```python
from build123d import *

# Parameters (mm, degrees)
SKETCH1_W           = 79.375
SKETCH1_H           = 82.55
SKETCH1_R           = 32.54375
BOSS_EXTRUDE1_DEPTH = 4.7625
SKETCH2_R           = 1.5875
CUT_EXTRUDE1_DEPTH  = 12.7
SKETCH3_W           = 12.7
SKETCH3_H           = 6.35
CUT_EXTRUDE2_DEPTH  = 10.525
FILLET1_R           = 1.5875


with BuildPart() as part:
    # Sketch1 → Boss-Extrude1 (new body, symmetric)
    with BuildSketch(Plane(origin=(0, 0, 0), x_dir=(1, 0, 0), z_dir=(0, 1, 0))):
        Rectangle(SKETCH1_W, SKETCH1_H)
        Circle(SKETCH1_R, mode=Mode.SUBTRACT)
    extrude(amount=BOSS_EXTRUDE1_DEPTH, both=True)

    # Sketch2 → Cut-Extrude1 (cut)
    with BuildSketch(Plane.ZY.offset(39.6875)):
        with Locations((-22.225, 0)):
            Circle(SKETCH2_R)
        with Locations((22.225, 0)):
            Circle(SKETCH2_R)
    cut_extrude1 = extrude(amount=-CUT_EXTRUDE1_DEPTH, mode=Mode.SUBTRACT)

    # Mirror1: Cut-Extrude1 across plane
    add(cut_extrude1.mirror(Plane(origin=(0, 0, 0), x_dir=(0, 0, 1), z_dir=(1, 0, 0))), mode=Mode.SUBTRACT)

    # Sketch3 → Cut-Extrude2 (cut, through all)
    with BuildSketch(Plane(origin=(34.925, 4.7625, 0), x_dir=(0, 0, -1), z_dir=(0, -1, 0))):
        with Locations((34.925, 1.5875)):
            Rectangle(SKETCH3_W, SKETCH3_H)
    extrude(amount=CUT_EXTRUDE2_DEPTH, mode=Mode.SUBTRACT)

    # Fillet1
    fillet1_edges = [part.edges().sort_by_distance(p)[0] for p in [
        (33.3375, 0, -28.575),
    ]]
    fillet(fillet1_edges, radius=FILLET1_R)


solid = part.part
```
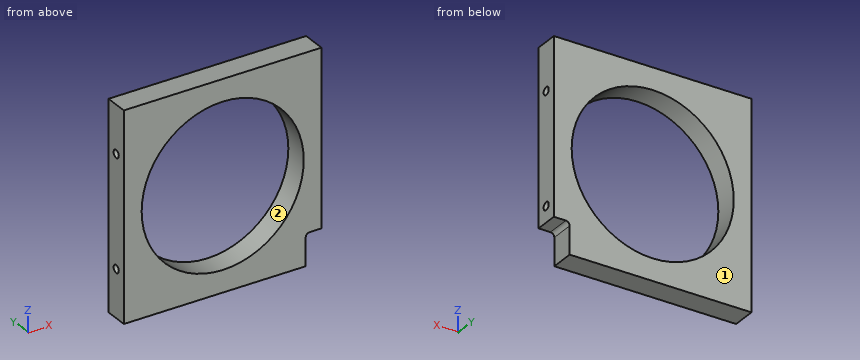
Geometry check sheet. Reference: the model listing, model coordinates, mm. Face numbers are marked on the shaded views. Coordinates: 2 decimals unless noted, no trailing zeros. Loops run counter-clockwise (first coordinate to the right, second up) from the corner with the lowest first, then second, coordinate; pieces in that order, holes last.
Item 1: Release check for a two-part mould opening along Z. For the marked faces 1 and 2 record: released by +Z, released by -Z, zero draft, split by the parting line, or undercut.
Item 2: Sectioned sample at A-A, the plane z = 0. Record the boundary of the cut face in (x, y), then the cut area to 3 significant figures.
Item 3: Thickness scan on line 1 (X direction, y = 2.75, z = 0); line 2 (Z direction, x = 0, y = -1.5) (3 decimals); line 3 (Z direction, x = -4, y = -1.25) (3 decimals). Record the ranges inside material, lowest first.
Item 4: Sectioned sample at B-B, the plane x = 7.5. Record the boundary of the cut face in (y, z) (1 decimal).
Item 5: Sectioned sample at D-D, the plane x = -34. Record the boundary of the cut face in (y, z) (1 decimal).
Item 6: Sectioned sample at C-C, the plane y = 0. Record the boundary of the cut face in (x, z) (1 decimal).
Item 7: Go/stop test with flat-tipped pins: pin 1 Ø1 at (y, z) = (-0.5, -21.5) entering from +X; pin 2 Ø5 at (x, y) = (37.5, -0.5) entering from -Z (3 decimals); pin 3 Ø1.6 at (y, z) = (0.5, 22.5) entering from -X. Record where each tip stops, or that it passes through.
Check result:
1. face 1: zero draft
1. face 2: undercut
2. outline: (-39.69, -4.76) - (-32.54, -4.76) - (-32.54, 4.76) - (-39.69, 4.76) - close; (32.54, -4.76) - (39.69, -4.76) - (39.69, 4.76) - (32.54, 4.76) - close
2. area: 136 mm2
3. line 1: x = -39.69 to -32.54, 32.54 to 39.69
3. line 2: z = -41.275 to -32.544, 32.544 to 41.275
3. line 3: z = -41.275 to -32.297, 32.297 to 41.275
4. outline: (-4.8, -41.3) - (4.8, -41.3) - (4.8, -31.7) - (-4.8, -31.7) - close; (-4.8, 31.7) - (4.8, 31.7) - (4.8, 41.3) - (-4.8, 41.3) - close
5. outline: (-4.8, -41.3) - (4.8, -41.3) - (4.8, 41.3) - (-4.8, 41.3) - close; hole circle Ø3.2 at (0, -22.2); hole circle Ø3.2 at (0, 22.2)
6. outline: (-39.7, -41.3) - (33.3, -41.3) - (33.3, -30.2) arc R1.6 cw to (34.9, -28.6) - (39.7, -28.6) - (39.7, -23.8) - (27, -23.8) - (27, -20.6) - (39.7, -20.6) - (39.7, 20.6) - (27, 20.6) - (27, 23.8) - (39.7, 23.8) - (39.7, 41.3) - (-39.7, 41.3) - (-39.7, 23.8) - (-27, 23.8) - (-27, 20.6) - (-39.7, 20.6) - (-39.7, -20.6) - (-27, -20.6) - (-27, -23.8) - (-39.7, -23.8) - close; hole circle Ø65.1 at (0, 0)
7. pin 1: stops at x = 26.99
7. pin 2: stops at z = -28.575
7. pin 3: stops at x = -26.99
